Check sheet for the modelled part. Datum: model origin and axes. Units: mm. A direction names the side the tool comes from. Give positions to 0.01 mm unless a question says otherwise; leave off trailing zeros. Loops run counter-clockwise (first coordinate to the right, second up) from the corner with the lowest first, then second, coordinate; pieces in that order, holes last. Notation, with made-up numbers: (-26.5, -13.75) - (-9.5, -13.75) arc R24 ccw to (-9.5, 13.25) - close; hole circle Ø2 at (13, 49). An arc over 180 degrees is marked (long way). Answer in a Markdown table with one row per item. Add a question column.
(1) Sectioned sample at D-D on y = -15.25. Enter the section's corners in (x, z).
(2) Draft check along Y on faces 4 (the face through (0.533, -24.649, 28.167)), 5 (the face through (1, -9, 29.996)), 6 (the face through (0.533, -15.461, 17.296)). Enter one of: released by +Y, released by -Y, zero draft, split by the parting line, or undercut.
(3) Sectioned sample at A-A on z = 25.25. Enter the section's corners in (x, y).
(4) Sectioned sample at B-B on x = -13. Enter the section's corners in (y, z) (3 decimals).
(5) Set-up check for faces 1 (the face through (1, -9, 29.742)), 2 (the face through (1, -12.356, 25)), 3 (the face through (1, -18.96, 24)): record each of +Z, -Z, +X, -X, +Y, -Y from which the full face is reachable in a straight line by a thin tool's end or side.
(6) Thickness scan on L1, parallel to Y at x = 2, z = 25.75; L2, parallel to Y at x = 32, z = 28.5; L3, parallel to Y at x = -11, z = 26.75. Record the ranges inside material, lowest first.
(7) Go/stop test with flat-tipped pins: P1, Ø1.8, axis at x = -9, y = -9, coming from the -Z side; P2, Ø3, axis at x = -14.5, z = 25.5, coming from the -Y side; P3, Ø3, axis at x = -15, y = -19.5, coming from the +Z side; P4, Ø2, axis at x = -0.5, y = -17, coming from the -Z side. Record where each tip stops, or that it passes through.
(8) Sectioned sample at C-C on y = -10.25. Enter the section's corners in (x, z).
from build123d import *

# Parameters (mm, degrees)
F1_DEPTH = 38.1


with BuildPart() as f1:
    # F0 (on Right) → F1 (new body, symmetric)
    with BuildSketch(Plane.YZ):
        with BuildLine():
            Line((-20.306327, 29.995541), (-22.820927, 29.995541))
            Line((-22.820927, 29.995541), (-26.529327, 26.287141))
            Line((-26.529327, 26.287141), (-26.349722, 26.107536))
            Line((-26.349722, 26.107536), (-22.715717, 29.741541))
            Line((-22.715717, 29.741541), (-20.306327, 29.741541))
            ThreePointArc((-20.306327, 29.741541), (-19.35442, 29.347248), (-18.960127, 28.395341))
            Line((-18.960127, 28.395341), (-18.960127, 20.470541))
            ThreePointArc((-18.960127, 20.470541), (-15.531127, 17.041541), (-12.102127, 20.470541))
            Line((-12.102127, 20.470541), (-12.102127, 29.741541))
            Line((-12.102127, 29.741541), (-6.209327, 29.741541))
            Line((-6.209327, 29.741541), (-6.209327, 29.995541))
            Line((-6.209327, 29.995541), (-12.356127, 29.995541))
            Line((-12.356127, 29.995541), (-12.356127, 20.470541))
            ThreePointArc((-12.356127, 20.470541), (-15.531127, 17.295541), (-18.706127, 20.470541))
            Line((-18.706127, 20.470541), (-18.706127, 28.395341))
            ThreePointArc((-18.706127, 28.395341), (-19.174815, 29.526853), (-20.306327, 29.995541))
        make_face()
    extrude(amount=F1_DEPTH, both=True)


solid = f1.part
Reply:
| question | item | result |
|---|---|---|
| 1 | outline | (-38.1, 17.05) - (38.1, 17.05) - (38.1, 17.31) - (-38.1, 17.31) - close |
| 2 | face 4 | released by -Y |
| 2 | face 5 | zero draft |
| 2 | face 6 | undercut |
| 3 | outline | (-38.1, -18.96) - (38.1, -18.96) - (38.1, -18.71) - (-38.1, -18.71) - close; (-38.1, -12.36) - (38.1, -12.36) - (38.1, -12.1) - (-38.1, -12.1) - close |
| 4 | outline | (-26.529, 26.287) - (-26.35, 26.108) - (-22.716, 29.742) - (-20.306, 29.742) arc R1.346 cw to (-18.96, 28.395) - (-18.96, 20.471) arc R3.429 ccw to (-12.102, 20.471) - (-12.102, 29.742) - (-6.209, 29.742) - (-6.209, 29.996) - (-12.356, 29.996) - (-12.356, 20.471) arc R3.175 cw to (-18.706, 20.471) - (-18.706, 28.395) arc R1.6 ccw to (-20.306, 29.996) - (-22.821, 29.996) - close |
| 5 | face 1 | -Z, +X, -X, +Y |
| 5 | face 2 | +Z, +X, -X |
| 5 | face 3 | -Z, +X, -X |
| 6 | L1 | -18.96 to -18.71, -12.36 to -12.1 |
| 6 | L2 | -24.32 to -23.96, -18.96 to -18.71, -12.36 to -12.1 |
| 6 | L3 | -26.07 to -25.71, -18.96 to -18.71, -12.36 to -12.1 |
| 7 | P1 | z = 29.74 |
| 7 | P2 | y = -26.53 |
| 7 | P3 | z = 30 |
| 7 | P4 | z = 17.07 |
| 8 | outline | (-38.1, 29.74) - (38.1, 29.74) - (38.1, 30) - (-38.1, 30) - close |
